Read the model definition and answer for the solid it produces. Units are mm, in the model's axes. A direction names the side the tool comes from. Give positions to 0.01 mm unless a question says otherwise; leave off trailing zeros. Loops run counter-clockwise (first coordinate to the right, second up) from the corner with the lowest first, then second, coordinate; pieces in that order, holes last. Notation, with made-up numbers: (25, -5) -> (77, -5) arc R23 cw to (77, 25) -> close; hole circle Ø1 at (1, -22). An arc over 180 degrees is marked (long way). One line per item, written item: value. Start each with the question number.
from build123d import *

# Parameters (mm, degrees)
F1_DEPTH       = 6.35
F3_D           = 5
F3_CSINK_D     = 9.1186
F3_CSINK_ANGLE = 82
F4_R           = 2.54


with BuildPart() as f1:
    # F0 (on Top) → F1 (new body, symmetric)
    with BuildSketch(Plane.XY):
        with BuildLine():
            ThreePointArc((-1.357143, 12.627279), (9.447902, -8.486881), (-12.7, 0))
            Line((-12.7, 0), (-12.7, 38.1))
            Line((-12.7, 38.1), (-15.875, 38.1))
            Line((-15.875, 38.1), (-15.875, 0))
            ThreePointArc((-15.875, 0), (11.809878, -10.608601), (-1.696429, 15.784098))
            ThreePointArc((-1.696429, 15.784098), (-6.61844, 17.373786), (-8.725, 22.097737))
            Line((-8.725, 22.097737), (-8.725, 38.1))
            Line((-8.725, 38.1), (-11.9, 38.1))
            Line((-11.9, 38.1), (-11.9, 22.097737))
            ThreePointArc((-11.9, 22.097737), (-8.74016, 15.011811), (-1.357143, 12.627279))
        make_face()
    extrude(amount=F1_DEPTH, both=True)

    # F3 (through all)
    with Locations(Plane.YZ.offset(-8.725)):
        with Locations((30.098869, 0)):
            CounterSinkHole(F3_D / 2, F3_CSINK_D / 2, counter_sink_angle=F3_CSINK_ANGLE)

    # F4
    f4_edges = [f1.edges().sort_by_distance(p)[0] for p in [
        (-14.2875, 38.1, 6.35),
        (-10.3125, 38.1, -6.35),
        (-14.2875, 38.1, -6.35),
        (-10.3125, 38.1, 6.35),
    ]]
    fillet(f4_edges, radius=F4_R)


solid = f1.part
Item 1: Consider L1, parallel to X at y = 0, z = 3 (3 decimals); L2, parallel to X at y = 24, z = 5.25 (3 decimals); L3, parallel to Y at x = -10, z = 2.5. Determine where each line is inside the solid, lowest interval first. Write a range as [from, to].
Item 2: Section A-A, the plane x = 0 is taken. Determine the outline of the cut face in (y, z) (3 decimals), plus the area to 3 significant figures.
Item 3: Flat-ended cylindrical pins translate along their axes: pin 1 (4 mm diameter, centred on y = 32, z = -3, fed in from +X) (3 decimals); pin 2 (3 mm diameter, centred on x = 7, z = 0.5, fed in from +Y). Find the tip coordinate at first contact, or state that the pin passes through.
Item 4: For faces 1 (the cylindrical face through (-6.56, 17.32, 0.09)), 2 (the cylindrical face through (11.445, -11.001, 0.089)), determine the directions among +Z, -Z, +X, -X, +Y, -Y from which every point of the face is accessible in a straight line to the end or side of a thin tool.
Item 5: Section B-B, the plane z = 0 is taken. Determine the outline of the cut face in (x, y) (3 decimals).
Item 6: Section C-C, the plane y = 19 is taken. Determine the outline of the cut face in (x, z) (3 decimals), plus the area to 3 significant figures.
Item 7: Determine the mould class of faces 3 (the cylindrical face through (9.7, -8.2, 0.1)), 4 (the flat face through (-8.725, 26, 3)), 5 (the cylindrical face through (-14.31, 37.376, 5.586)), 6 (the cylindrical face through (-8.823, 15.087, 0.089)) for opening direction Y: pulls with the +Y half, pulls with the -Y half, needs draft (parallel to the pull), parting line crosses it, or undercut.
Computed values:
1. L1: [-15.875, -12.7], [12.7, 15.875]
1. L2: [-15.875, -12.7], [-11.9, -8.725]
1. L3: [-12.33, -7.83], [16.39, 27.72], [32.48, 38.1]
2. outline: (-15.875, -6.35) -> (-12.7, -6.35) -> (-12.7, 6.35) -> (-15.875, 6.35) -> close; (12.7, -6.35) -> (15.875, -6.35) -> (15.875, 6.35) -> (12.7, 6.35) -> close
2. area: 80.6 mm²
3. pin 1: x = -8.725
3. pin 2: y = 14.89
4. face 1: +Z, -Z, +Y
4. face 2: +Z, -Z
5. outline: (-15.875, 0) arc R15.875 ccw (long way) to (-1.696, 15.784) arc R6.35 cw to (-8.725, 22.098) -> (-8.725, 25.54) -> (-11.094, 27.599) -> (-11.9, 27.599) -> (-11.9, 22.098) arc R9.525 ccw to (-1.357, 12.627) arc R12.7 cw (long way) to (-12.7, 0) -> (-12.7, 27.599) -> (-15.875, 27.599) -> close; (-15.875, 32.599) -> (-12.7, 32.599) -> (-12.7, 38.1) -> (-15.875, 38.1) -> close; (-11.9, 32.599) -> (-11.094, 32.599) -> (-8.725, 34.658) -> (-8.725, 38.1) -> (-11.9, 38.1) -> close
6. outline: (-15.875, -6.35) -> (-12.7, -6.35) -> (-12.7, 6.35) -> (-15.875, 6.35) -> close; (-11.382, -6.35) -> (-7.918, -6.35) -> (-7.918, 6.35) -> (-11.382, 6.35) -> close
6. area: 84.3 mm²
7. face 3: undercut
7. face 4: needs draft
7. face 5: pulls with the +Y half
7. face 6: undercut
